```python
from build123d import *

# Parameters (mm, degrees)
SKETCH008_R         = 1.25
SKETCH009_R         = 3
SKETCH006_R         = 1.25
SKETCH007_R         = 3
SKETCH004_R         = 1.5
SKETCH005_R         = 3
SKETCH002_R         = 1.5
SKETCH003_R         = 3
PAD_DEPTH           = 2
SKETCH001_R         = 1.5
POCKET_DEPTH        = 2.001
LINEARPATTERN_COUNT = 4
LINEARPATTERN_PITCH = 20
FILLET_R            = 1.5


with BuildPart() as loft003:
    # Sketch008 → Loft003 section 0
    with BuildSketch(Plane.XY):
        with Locations((35, -46)):
            Circle(SKETCH008_R)
    # Sketch009 → Loft003 section 1
    with BuildSketch(Plane.XY.offset(2)):
        with Locations((35, -46)):
            Circle(SKETCH009_R)
    loft(ruled=True)


with BuildPart() as loft002:
    # Sketch006 → Loft002 section 0
    with BuildSketch(Plane.XY):
        with Locations((35, 46)):
            Circle(SKETCH006_R)
    # Sketch007 → Loft002 section 1
    with BuildSketch(Plane.XY.offset(2)):
        with Locations((35, 46)):
            Circle(SKETCH007_R)
    loft(ruled=True)


with BuildPart() as loft001:
    # Sketch004 → Loft001 section 0
    with BuildSketch(Plane.XY):
        with Locations((-35, -46)):
            Circle(SKETCH004_R)
    # Sketch005 → Loft001 section 1
    with BuildSketch(Plane.XY.offset(2)):
        with Locations((-35, -46)):
            Circle(SKETCH005_R)
    loft(ruled=True)


with BuildPart() as loft_body:
    # Sketch002 → Loft section 0
    with BuildSketch(Plane.XY):
        with Locations((-35, 46)):
            Circle(SKETCH002_R)
    # Sketch003 → Loft section 1
    with BuildSketch(Plane.XY.offset(2)):
        with Locations((-35, 46)):
            Circle(SKETCH003_R)
    loft(ruled=True)


with BuildPart() as cut003:
    # Sketch → Pad (new body)
    with BuildSketch(Plane.XY):
        Polygon((-41.5, -50), (-41.5, -40.5), (-39.5, -40.5), (-39.5, -29.5), (-50, -29.5), (-50, -20.5), (-39.5, -20.5), (-39.5, -9.5), (-50, -9.5), (-50, -0.5), (-39.5, -0.5), (-39.5, 10.5), (-50, 10.5), (-50, 19.5), (-39.5, 19.5), (-39.5, 30.5), (-50, 30.5), (-50, 39.5), (-41.5, 39.5), (-41.5, 50), (41.5, 50), (41.5, 40.5), (39.5, 40.5), (39.5, 29.5), (50, 29.5), (50, 20.5), (39.5, 20.5), (39.5, 9.5), (50, 9.5), (50, 0.5), (39.5, 0.5), (39.5, -10.5), (50, -10.5), (50, -19.5), (39.5, -19.5), (39.5, -30.5), (50, -30.5), (50, -39.5), (41.5, -39.5), (41.5, -50), align=None)
    extrude(amount=PAD_DEPTH)

    # Sketch001 → Pocket (cut, through all)
    with BuildSketch(Plane.XY.offset(2)):
        with Locations((-46.75, -25)):
            Circle(SKETCH001_R)
        with Locations((46.75, -35)):
            Circle(SKETCH001_R)
    pocket = extrude(amount=-POCKET_DEPTH, mode=Mode.SUBTRACT)

    # LinearPattern: Pocket ×4
    with Locations(*[(0, i * LINEARPATTERN_PITCH, 0) for i in range(1, LINEARPATTERN_COUNT)]):
        add(pocket, mode=Mode.SUBTRACT)

    # Fillet
    fillet_edges = [cut003.edges().sort_by_distance(p)[0] for p in [
        (50, -39.5, 1),
        (-50, -29.5, 1),
        (50, -30.5, 1),
        (-50, -20.5, 1),
        (50, -19.5, 1),
        (-50, -9.5, 1),
        (50, -10.5, 1),
        (-50, -0.5, 1),
        (50, 0.5, 1),
        (-50, 10.5, 1),
        (50, 9.5, 1),
        (-50, 19.5, 1),
        (50, 20.5, 1),
        (-50, 30.5, 1),
        (50, 29.5, 1),
        (-50, 39.5, 1),
    ]]
    fillet(fillet_edges, radius=FILLET_R)

    # Cut: cut Loft body
    add(loft_body.part, mode=Mode.SUBTRACT)

    # Cut001: cut Loft001
    add(loft001.part, mode=Mode.SUBTRACT)

    # Cut002: cut Loft002
    add(loft002.part, mode=Mode.SUBTRACT)

    # Cut003: cut Loft003
    add(loft003.part, mode=Mode.SUBTRACT)


solid = cut003.part
```
Here's how the part is built. I have some questions about the finished solid (model axes, mm). Coordinates: 2 decimals unless noted, no trailing zeros. Order: outer loops, then holes, each group sorted by start corner. A loop starts at its lowest first (then second) coordinate and runs counter-clockwise, first axis right, second up. Notation, with made-up numbers: M 81.25,88 L 87.25,88 A28 cw 87.25,116 Z; hole C 79.5,8 d5. An arc over 180 degrees is marked long. Answer as a JSON object with one key per item and string values. Group by question number.
(1) For pin 1 (0.6 mm diameter, centred on y = -47, z = 1.5, fed in from +X); pin 2 (1 mm diameter, centred on x = -45.5, z = 1.5, fed in from +Y); pin 3 (2.5 mm diameter, centred on x = 46.75, y = -35, fed in from +Z); pin 4 (1 mm diameter, centred on y = 39.5, z = 0.5, fed in from -X), each with a flat end and sliding along its axis, tell me the tip position at first contact or that it passes through.
(2) Suppose I cut it at C-C, the plane x = 46.75. State how many separate pieces and enclosed holes the cut face has, then the cut area to 3 significant figures.
(3) If we mould it in two halves opening along X, with no side actions, what happens to faces 1 (the face through (45.64, 26.01, 1.01)), 2 (the face through (1, 1, 2))? For each: released by +X, released by -X, zero draft, split by the parting line, or undercut.
(4) I need wall thicknesses on probe 1 along X at (y, z) = (-27.5, 0.8); probe 2 along X at (y, z) = (42.5, 1.1). Which ranges of each line are inside material? Lowest first, please.
(5) Suppose I cut it at B-B, the plane x = -35. Please give me the cut outline in (y, z).
(6) Suppose I cut it at A-A, the plane y = 15. Please give me the cut outline in (x, z), then the cut area to 3 significant figures.
Values found:
{
 "1": {"pin 1": "stops at x = 41.5", "pin 2": "stops at y = 39.5", "pin 3": "passes through", "pin 4": "stops at x = -49.62"},
 "2": {"separate pieces": "8", "enclosed holes": "0", "area": "48.0 mm^2"},
 "3": {"face 1": "undercut", "face 2": "zero draft"},
 "4": {"probe 1": "x = -50 to 39.5", "probe 2": "x = -41.5 to 41.5"},
 "5": {"outline": "M -50,0 L -47.5,0 L -49,2 L -50,2 Z; M -44.5,0 L 44.5,0 L 43,2 L -43,2 Z; M 47.5,0 L 50,0 L 50,2 L 49,2 Z"},
 "6": {"outline": "M -50,0 L -48.25,0 L -48.25,2 L -50,2 Z; M -45.25,0 L 39.5,0 L 39.5,2 L -45.25,2 Z", "area": "173 mm^2"}
}
